from build123d import *

# Parameters (mm, degrees)
CROQUIS1_R              = 7.5
SALIENTE_EXTRUIR1_DEPTH = 15
CROQUIS2_R              = 6
SALIENTE_EXTRUIR2_DEPTH = 80
CROQUIS4_R              = 7.5
SALIENTE_EXTRUIR3_DEPTH = 5
SALIENTE_EXTRUIR4_DEPTH = 5
CROQUIS7_R              = 5.35
SALIENTE_EXTRUIR6_DEPTH = 8.39
CROQUIS8_R              = 5.641199124
SALIENTE_EXTRUIR7_DEPTH = 10
CROQUIS9_R              = 1.540513395
SALIENTE_EXTRUIR8_DEPTH = 20


with BuildPart() as part:
    # Croquis1 → Saliente-Extruir1 (new body)
    with BuildSketch(Plane.XY):
        with Locations((-11.670259109, 4.990389294)):
            Circle(CROQUIS1_R)
    extrude(amount=SALIENTE_EXTRUIR1_DEPTH)

    # Croquis2 → Saliente-Extruir2 (add)
    with BuildSketch(Plane.XY.offset(15)):
        with Locations((-11.670259109, 4.990389294)):
            Circle(CROQUIS2_R)
    extrude(amount=SALIENTE_EXTRUIR2_DEPTH)

    # Croquis4 → Saliente-Extruir3 (add)
    with BuildSketch(Plane.XY.offset(95)):
        with Locations((-11.658111308, 5.002537095)):
            Circle(CROQUIS4_R)
    extrude(amount=SALIENTE_EXTRUIR3_DEPTH)

    # Croquis5 → Saliente-Extruir4 (add)
    with BuildSketch(Plane.XY.offset(100)):
        Polygon((-7.518768123, 4.990389294), (-7.518768123, 11.066839741), (-15.877144731, 11.066839741), (-15.877144731, -1.023256523), (-7.518768123, -1.023256523), align=None)
    extrude(amount=SALIENTE_EXTRUIR4_DEPTH)

    # Croquis7 → Saliente-Extruir6 (add)
    with BuildSketch(Plane.XY.offset(105)):
        with Locations((-11.670259109, 4.990389294)):
            Circle(CROQUIS7_R)
    extrude(amount=SALIENTE_EXTRUIR6_DEPTH)

    # Croquis8 → Saliente-Extruir7 (add)
    with BuildSketch(Plane(origin=(0, 0, 0), x_dir=(-1, 0, 0), z_dir=(0, 0, -1))):
        with Locations((11.670259109, 4.990389294)):
            Circle(CROQUIS8_R)
    extrude(amount=SALIENTE_EXTRUIR7_DEPTH)

    # Croquis9 → Saliente-Extruir8 (add)
    with BuildSketch(Plane(origin=(0, 0, -10), x_dir=(-1, 0, 0), z_dir=(0, 0, -1))):
        with Locations((11.670259109, 4.990389294)):
            Circle(CROQUIS9_R)
    extrude(amount=SALIENTE_EXTRUIR8_DEPTH)


solid = part.part
Input: part model. Units: mm. Frame: model coordinates. A direction names the side the tool comes from. Coordinates: 2 decimals unless noted, no trailing zeros. Order: outer loops, then holes, each group sorted by start corner. A loop starts at its lowest first (then second) coordinate and runs counter-clockwise, first axis right, second up. Notation, with made-up numbers: M 1,-19 L 27,-19 A18 cw 27,-15 Z; hole C -17.5,65 d2. An arc over 180 degrees is marked long. Write item = value, one per line. Start each with the question number.
(1) Reachability of faces 1 (the flat face through (-7.519, 5, 102)), 2 (the flat face through (-15.877, 5, 102)), 3 (the flat face through (-11.8, -0.6, 105)), 4 (the cylindrical face through (-12.5, 6.29, -19.86)), 5 (the cylindrical face through (-16.4, 1.3, 54.4)) from +Z, -Z, +X, -X, +Y, -Y: full face, straight path, thin tool, end or side. Return the list, or none.
(2) Line query: line 1 along Z through (x, y) = (-17.75, 0.75); line 2 along Z through (x, y) = (-14, 9.5); line 3 along Z through (x, y) = (-7, 8). Output: solid intervals per line, ascending. Write a range as [from, to].
(3) Section A-A on x = -12. Output: boundary loops of the cut face in (y, z).
(4) First-contact query: P1, Ø4, axis at y = 6.5, z = 103.5, coming from the +X side; P2, Ø5.5, axis at y = 6.5, z = 103.5, coming from the -X side; P3, Ø5.5, axis at x = -11.5, y = 2.5, coming from the -Z side; P4, Ø1.3, axis at x = -16.5, y = 5, coming from the -Z side. Flat tips, straight axial feed; report the tip coordinate or a pass-through.
(5) Section C-C on z = 73. Output: boundary loops of the cut face in (x, y).
(6) Pull-direction query (Z, two-part tool) for faces 6 (the flat face through (-12, 5, -30)), 7 (the flat face through (-14, 11, 95)), 8 (the cylindrical face through (-12.647, 12.427, 7.395)); classes: released by +Z, released by -Z, zero draft, split by the parting line, or undercut.
(7) Section B-B on z = -2.5. Output: boundary loops of the cut face in (x, y), and give its area (4 significant figures).
Result set:
q1.face_1 = +X, +Y, -Y
q1.face_2 = -X, +Y, -Y
q1.face_3 = +Z, -Y
q1.face_4 = -Z
q1.face_5 = none
q2.line_1 = [0, 15], [95, 100]
q2.line_2 = [-10, 113.39]
q2.line_3 = [-10, 100]
q3.outline = M -2.5,0 L -0.64,0 L -0.64,-10 L 3.49,-10 L 3.49,-30 L 6.5,-30 L 6.5,-10 L 10.62,-10 L 10.62,0 L 12.48,0 L 12.48,15 L 10.98,15 L 10.98,95 L 12.49,95 L 12.49,100 L 11.07,100 L 11.07,105 L 10.33,105 L 10.33,113.39 L -0.35,113.39 L -0.35,105 L -1.02,105 L -1.02,100 L -2.49,100 L -2.49,95 L -1,95 L -1,15 L -2.5,15 Z
q4.P1 = -6.32
q4.P2 = -17.02
q4.P3 = -30
q4.P4 = -10
q5.outline = C -11.67,4.99 d12
q6.face_6 = released by -Z
q6.face_7 = undercut
q6.face_8 = zero draft
q7.outline = C -11.67,4.99 d11.28
q7.area = 100.0 mm²
